Design review of the part built by this model. Coordinates are the model's own, in mm. A direction names the side the tool comes from. Round coordinates to 2 decimals unless told otherwise and drop trailing zeros. Order: outer loops, then holes, each group sorted by start corner. A loop starts at its lowest first (then second) coordinate and runs counter-clockwise, first axis right, second up. Notation, with made-up numbers: (56, 17) - (74, 17) arc R11 ccw to (74, 34) - close; hole circle Ø7 at (-9, 4). An arc over 180 degrees is marked (long way). Write item = value, one per line.
Autodesk Inventor part; units mm, degrees
ref_plane "YZ Plane" through (0, 0, 0) normal (1, 0, 0) x (0, 1, 0)
ref_plane "XZ Plane" through (0, 0, 0) normal (0, 1, 0) x (-1, 0, 0)
ref_plane "XY Plane" through (0, 0, 0) normal (0, 0, 1) x (1, 0, 0)
sketch "Skizze1" plane through (0, 0, 0) normal (0, 1, 0) x (-1, 0, 0)
  circle A0 centre (0, 0) radius 7
  dimension "d0" = 14
extrude "Extrusion1" add sketch "Skizze1" along normal blind 24
sketch "Skizze2" plane through (0, 24, 0) normal (0, 1, 0) x (1, 0, 0)
  circle A0 centre (0, 0) radius 3.5
  dimension "d3" = 7
extrude "Extrusion2" add sketch "Skizze2" along normal blind 0.5
fillet "Rundung1" radius 0.5 1 edges at (-3.5, 24.5, 0)
sketch "Skizze3" plane through (0, 0, 0) normal (0, -1, 0) x (1, 0, 0)
  circle A0 centre (0, 0) radius 3.5
  circle A1 centre (0, 0) radius 5.4598
extrude "Extrusion3" add sketch "Skizze3" along normal blind 0.5 contours A0 | A1
properties part number "Li-Ion 14250"
Item 1: Insertion check: P1, Ø1.5, axis at y = 15, z = -1.5, coming from the +X side; P2, Ø4, axis at x = 5.5, y = 10.5, coming from the -Z side; P3, Ø5, axis at y = 22, z = 3, coming from the -X side. Each pin has a flat end and moves straight along its axis. Give the tip position at first contact, or say it passes through.
Data:
P1 = 6.96
P2 = -6.06
P3 = -6.98
Item 2: For line 1 along Y through (x, z) = (3.25, -5); line 2 along Y through (x, z) = (2.25, 3.5); line 3 along X through (y, z) = (2.25, -0.25), list the stretches that pass through material, from the lowest coordinate up. Write a range as [from, to].
Data:
line_1 = [0, 24]
line_2 = [-0.5, 24]
line_3 = [-7, 7]
Item 3: For faces 1 (the face through (-4, 0, -4)), 2 (the face through (-3, 24, -3)), 3 (the face through (0, 24.5, 0)), list the 3-axis set-ups (+Z, -Z, +X, -X, +Y, -Y) from which the entire face can be reached by the end or side of a thin tool; tool diameter is ignored.
Data:
face_1 = -Y
face_2 = +Y
face_3 = +Z, -Z, +X, -X, +Y
Item 4: Take a section at A-A, the plane y = 19.25. State the section outline as (x, z) points.
Data:
outline = circle Ø14 at (0, 0)
